Geometry check sheet. Reference: the model listing, model coordinates, mm. A direction names the side the tool comes from. Give positions to 0.01 mm unless a question says otherwise; leave off trailing zeros. Write each loop counter-clockwise with the first axis right and the second up, starting at its lowest first coordinate (ties: lowest second). Pieces come first, ordered by that corner, then holes. Notation, with made-up numbers: (79, 7.25) -> (112, 7.25) arc R31 ccw to (112, 31.25) -> close; hole circle Ø3 at (-14, 17). An arc over 180 degrees is marked (long way). One line per item, written item: value.
from build123d import *

# Parameters (mm, degrees)
F2_R      = 12
F0_R      = 22
F6_R      = 42
F6_R_2    = 20
F7_DEPTH  = 5
F5_R      = 20
F4_R      = 10
F9_R      = 5
F10_DEPTH = 5
F4_R_2    = 12
F11_DEPTH = 30
F12_R     = 32
F12_R_2   = 12
F13_DEPTH = 5
F14_R     = 5
F15_DEPTH = 5


with BuildPart() as f3:
    # F2 (on offset) → F3 section 0
    with BuildSketch(Plane.XY.offset(50)):
        Circle(F2_R)
    # F0 (on Top) → F3 section 1
    with BuildSketch(Plane.XY):
        Circle(F0_R)
    loft()

    # F6 (on face) → F7 (join)
    with BuildSketch(Plane(origin=(0, 0, 0), x_dir=(1, 0, 0), z_dir=(0, 0, -1))):
        Circle(F6_R)
        Circle(F6_R_2, mode=Mode.SUBTRACT)
    extrude(amount=-F7_DEPTH)

    # F5 (on face) → F8 section 0
    with BuildSketch(Plane(origin=(0, 0, 0), x_dir=(1, 0, 0), z_dir=(0, 0, -1))):
        Circle(F5_R)
    # F4 (on face) → F8 section 1
    with BuildSketch(Plane.XY.offset(50)):
        Circle(F4_R)
    loft(mode=Mode.SUBTRACT)

    # F9 (on face) → F10 (cut, through all)
    with BuildSketch(Plane(origin=(0, 0, 0), x_dir=(1, 0, 0), z_dir=(0, 0, -1))):
        with Locations((0, 30)):
            Circle(F9_R)
        with Locations((-25.9807621135, 15)):
            Circle(F9_R)
        with Locations((25.9807621135, 15)):
            Circle(F9_R)
        with Locations((25.9807621135, -15)):
            Circle(F9_R)
        with Locations((0, -30)):
            Circle(F9_R)
        with Locations((-25.9807621135, -15)):
            Circle(F9_R)
    extrude(amount=-F10_DEPTH, mode=Mode.SUBTRACT)

    # F4 (on face) → F11 (join)
    with BuildSketch(Plane.XY.offset(50)):
        Circle(F4_R_2)
        Circle(F4_R, mode=Mode.SUBTRACT)
    extrude(amount=F11_DEPTH)

    # F12 (on face) → F13 (join)
    with BuildSketch(Plane.XY.offset(80)):
        Circle(F12_R)
        Circle(F12_R_2, mode=Mode.SUBTRACT)
    extrude(amount=-F13_DEPTH)

    # F14 (on face) → F15 (cut, through all)
    with BuildSketch(Plane.XY.offset(80)):
        with Locations((0, 20)):
            Circle(F14_R)
        with Locations((-20, 0)):
            Circle(F14_R)
        with Locations((0, -20)):
            Circle(F14_R)
        with Locations((20, 0)):
            Circle(F14_R)
    extrude(amount=-F15_DEPTH, mode=Mode.SUBTRACT)


solid = f3.part
1) Sectioned sample at B-B on z = 63. Record the cut outline in (x, y), plus the area to 3 significant figures.
Verdict:
outline: circle Ø24 at (0, 0); hole circle Ø20 at (0, 0)
area: 138 mm^2
2) Sectioned sample at C-C on y = 0. Give the number of separate pieces and of enclosed holes in the cut face, plus the area to 3 significant figures.
Verdict:
separate pieces: 4
enclosed holes: 0
area: 625 mm^2
3) Tool access check on faces 1 (the cylindrical face through (28.288, -10.564, 2.465)), 2 (the flat face through (8.7, -19.3, 5)), 3 (the cylindrical face through (15, 0, 78)), 4 (the flat face through (18, -10, 0)). Record the directions out of +Z, -Z, +X, -X, +Y, -Y that give a thin tool (end or side, any length) a straight path to the whole face; none if there is none.
Verdict:
face 1: -Z
face 2: none
face 3: +Z
face 4: -Z, +X, -X, +Y, -Y
4) Mould release check, pull along X, two halves, no side actions. Record for faces 5 (the cylindrical face through (40.06, -12.62, 2.46)), 6 (the flat face through (7, 8, 80)), 7 (the cylindrical face through (-1.08, 34.88, 2.46)): released by +X, released by -X, zero draft, split by the parting line, or undercut.
Verdict:
face 5: split by the parting line
face 6: zero draft
face 7: undercut
5) Depth check by flat-ended pin: pin 1 Ø1.5 at (x, y) = (16, -15) entering from -Z; pin 2 Ø1.5 at (y, z) = (-3.5, 42) entering from +X; pin 3 Ø12 at (x, z) = (15.5, 67) entering from +Y; pin 4 Ø6 at (x, y) = (25.98, -15) entering from -Z. Enter the tip coordinate at first touch or a pass-through.
Verdict:
pin 1: z = 0
pin 2: x = 13.38
pin 3: y = 7.33
pin 4: z = 75
6) Sectioned sample at A-A on y = -28. Record the cut outline in (x, z), plus the area to 3 significant figures.
Verdict:
outline: (-31.3, 0) -> (-4.58, 0) -> (-4.58, 5) -> (-31.3, 5) -> close; (-15.49, 75) -> (15.49, 75) -> (15.49, 80) -> (-15.49, 80) -> close; (4.58, 0) -> (31.3, 0) -> (31.3, 5) -> (4.58, 5) -> close
area: 422 mm^2
7) Scan lines: probe 1 along Y at (x, z) = (0, 76.15); probe 2 along Y at (x, z) = (-20, 77); probe 3 along Z at (x, y) = (-15, 27.5). Record each from-to range of solid material in increasing order.
Verdict:
probe 1: -32 to -25, -15 to -10, 10 to 15, 25 to 32
probe 2: -24.98 to -5, 5 to 24.98
probe 3: 0 to 5, 75 to 80
